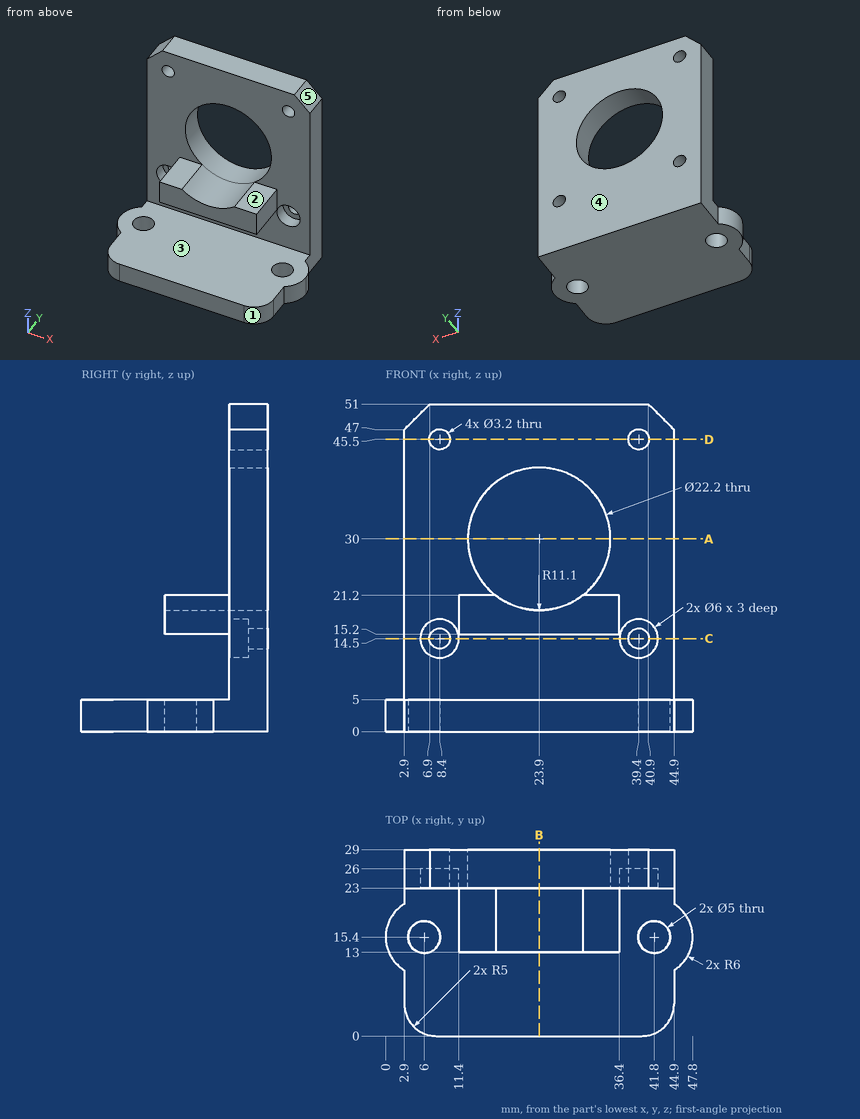
Could you check a few things on this drawing? It's one solid part, dimensions in mm from its lowest x, y, z. A direction names the side the tool comes from. Coordinates: 2 decimals unless noted, no trailing zeros. Order: outer loops, then holes, each group sorted by start corner. A loop starts at its lowest first (then second) coordinate and runs counter-clockwise, first axis right, second up. Notation, with made-up numbers: M 15,-40 L 31,-40 A22 cw 31,-7 Z; hole C 15,79 d6. An arc over 180 degrees is marked long. Use a Markdown table: item, result. Add a question column.
Q1. I want a section at C-C on z = 14.5. List the corners of the cut face in (x, y) for me, then the cut area to 3 significant figures.
Q2. If I drill on L1, parallel to Z at x = 8.4, y = 24.4; L2, parallel to Z at x = 8.4, y = 27.35; L3, parallel to Z at x = 15.5, y = 20.5, over which ranges is the centre line in solid material (lowest first)?
Q3. We'd pull the mould along Z, two halves only. Please class the marked faces 3, 4 and 5: pulls with the +Z half, pulls with the -Z half, needs draft (parallel to the pull), parting line crosses it, or undercut.
Q4. Which directions (+Z, -Z, +X, -X, +Y, -Y) give clear straight access to the entire face, cutting with the end or side of a thin tool? Please do the marked faces 1 and 2.
Q5. I want a section at A-A on z = 30. List the corners of the cut face in (x, y) for me.
Q6. I want a section at D-D on z = 45.5. List the corners of the cut face in (x, y) for me, then the cut area to 3 significant figures.
Q7. I'm going to push flat-ended pins straight in: pin 1 (7 mm diameter, centred on y = 23, z = 13.5, fed in from +X); pin 2 (1 mm diameter, centred on x = 31.5, z = 10.5, fed in from -Y); pin 3 (5.5 mm diameter, centred on y = 8.5, z = 3.5, fed in from -X). Where does each tip first touch, or does it pass through?
Q8. I want a section at B-B on x = 23.9. List the corners of the cut face in (y, z) for me.
Checked values:
| question | item | result |
|---|---|---|
| 1 | outline | M 2.9,23 L 5.4,23 L 5.4,26 L 6.8,26 L 6.8,29 L 2.9,29 Z; M 10,26 L 11.4,26 L 11.4,23 L 36.4,23 L 36.4,26 L 37.8,26 L 37.8,29 L 10,29 Z; M 41,26 L 42.4,26 L 42.4,23 L 44.9,23 L 44.9,29 L 41,29 Z |
| 1 | area | 197 mm² |
| 2 | L1 | 0 to 11.5, 17.5 to 43.9, 47.1 to 51 |
| 2 | L2 | 0 to 12.9, 16.1 to 43.9, 47.1 to 51 |
| 2 | L3 | 0 to 5, 15.2 to 21.2 |
| 3 | face 3 | undercut |
| 3 | face 4 | needs draft |
| 3 | face 5 | pulls with the +Z half |
| 4 | face 1 | +Z, -Z, +X, -Y |
| 4 | face 2 | +Z, +X, -X, -Y |
| 5 | outline | M 2.9,23 L 12.8,23 L 12.8,29 L 2.9,29 Z; M 35,23 L 44.9,23 L 44.9,29 L 35,29 Z |
| 6 | outline | M 2.9,23 L 6.8,23 L 6.8,29 L 2.9,29 Z; M 10,23 L 37.8,23 L 37.8,29 L 10,29 Z; M 41,23 L 44.9,23 L 44.9,29 L 41,29 Z |
| 6 | area | 214 mm² |
| 7 | pin 1 | x = 44.9 |
| 7 | pin 2 | y = 23 |
| 7 | pin 3 | x = 1.67 |
| 8 | outline | M 0,0 L 29,0 L 29,18.9 L 13,18.9 L 13,15.2 L 23,15.2 L 23,5 L 0,5 Z; M 23,41.1 L 29,41.1 L 29,51 L 23,51 Z |
